Autodesk Inventor part; units mm, degrees
ref_plane "YZ Plane" through (0, 0, 0) normal (1, 0, 0) x (0, 1, 0)
ref_plane "XZ Plane" through (0, 0, 0) normal (0, 1, 0) x (-1, 0, 0)
ref_plane "XY Plane" through (0, 0, 0) normal (0, 0, 1) x (1, 0, 0)
sketch "Sketch1" plane through (0, 0, 0) normal (0, 0, 1) x (1, 0, 0)
  spline S0 degree 3 poles (-8.9262, 55.5372) (-8.7839, 55.3802) (-8.4991, 55.0662) (-8.0852, 54.5835) (-7.6813, 54.0924) (-7.2889, 53.592) (-6.9084, 53.0826) (-6.5406, 52.5638) (-6.1865, 52.0357) (-5.8469, 51.4981) (-5.5231, 50.9508) (-5.2164, 50.3937) (-4.9286, 49.8267) (-4.6617, 49.2495) (-4.4187, 48.6617) (-4.2033, 48.0633) (-4.0539, 47.5547) (-3.9553, 47.1422) (-3.9241, 46.9325) (-3.9085, 46.8277) knots 0 0 0 0 0.063581 0.127162 0.190743 0.254324 0.317905 0.381486 0.445066 0.508647 0.572227 0.635807 0.699386 0.762964 0.826542 0.890117 0.953687 0.985476 1.017256 1.017256 1.017256 1.017256
  spline S1 degree 3 poles (-3.9085, 46.8277) (-3.8988, 46.6849) (-3.8795, 46.3993) (-3.8286, 45.9728) (-3.7545, 45.5498) (-3.6583, 45.1311) (-3.5319, 44.7205) (-3.3763, 44.3201) (-3.189, 43.9333) (-2.9645, 43.5666) (-2.7433, 43.2845) (-2.5493, 43.0739) (-2.3922, 42.9274) (-2.2262, 42.7911) (-2.0526, 42.6646) (-1.8686, 42.5537) (-1.678, 42.4548) (-1.4812, 42.3683) (-1.2769, 42.302) (-1.0697, 42.2449) (-0.8577, 42.21) (-0.6441, 42.187) (-0.3577, 42.1846) (0, 42.1894) (0.3577, 42.1846) (0.6441, 42.187) (0.8577, 42.21) (1.0697, 42.2449) (1.2769, 42.302) (1.4812, 42.3683) (1.678, 42.4548) (1.8686, 42.5537) (2.0526, 42.6646) (2.2262, 42.7911) (2.3922, 42.9274) (2.5493, 43.0739) (2.7433, 43.2845) (2.9645, 43.5666) (3.189, 43.9333) (3.3763, 44.3201) (3.5319, 44.7205) (3.6583, 45.1311) (3.7545, 45.5498) (3.8286, 45.9728) (3.8795, 46.3993) (3.8988, 46.6849) (3.9085, 46.8277) knots 0 0 0 0 0.04293 0.085861 0.12879 0.17172 0.214646 0.257562 0.300476 0.343394 0.386302 0.407769 0.429238 0.450698 0.472163 0.49363 0.515088 0.536554 0.558017 0.579478 0.600945 0.622403 0.64387 0.686802 0.729734 0.751201 0.772659 0.794126 0.815587 0.83705 0.858516 0.879974 0.901441 0.922906 0.944366 0.965835 0.987302 1.03021 1.073128 1.116042 1.158958 1.201884 1.244814 1.287743 1.330674 1.373604 1.373604 1.373604 1.373604
  spline S2 degree 3 poles (3.9085, 46.8277) (3.9241, 46.9325) (3.9553, 47.1422) (4.0539, 47.5547) (4.2033, 48.0633) (4.4187, 48.6617) (4.6617, 49.2495) (4.9286, 49.8267) (5.2164, 50.3937) (5.5231, 50.9508) (5.8469, 51.4981) (6.1865, 52.0357) (6.5406, 52.5638) (6.9084, 53.0826) (7.2889, 53.592) (7.6813, 54.0924) (8.0852, 54.5835) (8.4991, 55.0662) (8.7839, 55.3802) (8.9262, 55.5372) knots 0 0 0 0 0.03178 0.063568 0.127139 0.190714 0.254291 0.31787 0.381449 0.445029 0.508609 0.572189 0.63577 0.699351 0.762932 0.826513 0.890094 0.953675 1.017256 1.017256 1.017256 1.017256
  circle A0 centre (0, 0) radius 42.1875 construction
  circle A1 centre (0, 0) radius 46.9846 construction
  circle A2 centre (0, 0) radius 50 construction
  circle A3 centre (0, 0) radius 56.25
  point P0 (-8.5013, 55.0643)
  point P1 (-8.0869, 54.5821)
  point P2 (-7.6832, 54.0908)
  point P3 (-7.2909, 53.5905)
  point P4 (-6.9105, 53.081)
  point P5 (-6.5429, 52.5623)
  point P6 (-6.1889, 52.0341)
  point P7 (-5.8496, 51.4965)
  point P8 (-5.526, 50.9492)
  point P9 (-5.2196, 50.3921)
  point P10 (-4.9321, 49.825)
  point P11 (-4.6657, 49.2477)
  point P12 (-4.4233, 48.6599)
  point P13 (-4.2093, 48.0613)
  point P14 (-4.031, 47.4511)
  point P15 (-3.9598, 47.1413)
  point P16 (-3.8758, 46.3996)
  point P17 (-3.8247, 45.9733)
  point P18 (-3.7508, 45.5505)
  point P19 (-3.6533, 45.1324)
  point P20 (-3.527, 44.7221)
  point P21 (-3.371, 44.3223)
  point P22 (-3.1828, 43.9367)
  point P23 (-2.9576, 43.5713)
  point P24 (-2.6935, 43.2332)
  point P25 (-2.5474, 43.0758)
  point P26 (-2.3907, 42.9291)
  point P27 (-2.225, 42.7928)
  point P28 (-2.0509, 42.6672)
  point P29 (-1.8675, 42.5557)
  point P30 (-1.677, 42.4569)
  point P31 (-1.48, 42.3717)
  point P32 (-1.2764, 42.3036)
  point P33 (-1.069, 42.2486)
  point P34 (-0.8574, 42.212)
  point P35 (-0.6439, 42.1905)
  point P36 (-0.4293, 42.1857)
  point P37 (0, 42.1875)
  point P38 (0.4293, 42.1857)
  point P39 (0.6439, 42.1905)
  point P40 (0.8574, 42.212)
  point P41 (1.069, 42.2486)
  point P42 (1.2764, 42.3036)
  point P43 (1.48, 42.3717)
  point P44 (1.677, 42.4569)
  point P45 (1.8675, 42.5557)
  point P46 (2.0509, 42.6672)
  point P47 (2.225, 42.7928)
  point P48 (2.3907, 42.9291)
  point P49 (2.5474, 43.0758)
  point P50 (2.6935, 43.2332)
  point P51 (2.9576, 43.5713)
  point P52 (3.1828, 43.9367)
  point P53 (3.371, 44.3223)
  point P54 (3.527, 44.7221)
  point P55 (3.6533, 45.1324)
  point P56 (3.7508, 45.5505)
  point P57 (3.8247, 45.9733)
  point P58 (3.8758, 46.3996)
  point P59 (3.9598, 47.1413)
  point P60 (4.031, 47.4511)
  point P61 (4.2093, 48.0613)
  point P62 (4.4233, 48.6599)
  point P63 (4.6657, 49.2477)
  point P64 (4.9321, 49.825)
  point P65 (5.2196, 50.3921)
  point P66 (5.526, 50.9492)
  point P67 (5.8496, 51.4965)
  point P68 (6.1889, 52.0341)
  point P69 (6.5429, 52.5623)
  point P70 (6.9105, 53.081)
  point P71 (7.2909, 53.5905)
  point P72 (7.6832, 54.0908)
  point P73 (8.0869, 54.5821)
  point P74 (8.5013, 55.0643)
extrude "Extrusion1" add sketch "Sketch1" against normal blind 16
extrude "Extrusion2" cut sketch "Sketch1" against normal through all contours A3 S2 S1 S0 picked at (0.9155, 51.5438)
pattern_circular "Circular Pattern1" count 16 over 360 about axis through (0, 0, 0) along (0, 0, -1) of "Extrusion2"
sketch "Measuring" plane through (0, 0, -16) normal (0, 0, -1) x (-1, 0, 0)
  circle A0 centre (0, 0) radius 56.25
  circle A1 centre (0, 0) radius 50
  circle A2 centre (73.063, 68.2774) radius 50 construction
  line L0 (27.9744, 52.4494) -> (54.2214, 24.3627) construction
  line L1 (41.0979, 38.406) -> (73.063, 68.2774) construction
  dimension "d37" = 100
  dimension "d45" = 6.25
  dimension "d46" = 100
  dimension "d47" = 43.75
sketch "Sketch11" plane through (0, 0, 0) normal (1, 0, 0) x (0, 1, 0)
  line L0 (13.8864, 0) -> (-13.8864, 0) construction
  line L1 (-13.8864, 0) -> (-13.8864, -7) construction
  line L2 (-13.8864, -7) -> (13.8864, -7) construction
  line L3 (13.8864, -7) -> (13.8864, 0) construction
  circle A0 centre (0, -3.5) radius 1.5 construction
  line L4 (-1.3941, -2) -> (1.3941, -2) construction
  line L5 (-3.9085, -16) -> (3.9085, -16) construction
  line L6 (-67.1444, 3.8787) -> (73.9482, 3.8787)
  line L7 (73.9482, 3.8787) -> (73.9482, -7)
  line L8 (73.9482, -7) -> (-67.1444, -7)
  line L9 (-67.1444, -7) -> (-67.1444, 3.8787)
  point P0 (0, 0)
  point P1 (0, 0)
  point P2 (-13.8864, -3.5)
  point P3 (0, -2)
  dimension "d48" = 3
  dimension "d49" = 2
  dimension "d50" = 9
  dimension "d58" = 7
extrude "Thinner" cut sketch "Sketch11" against normal through all both and the other way through all
sketch "Sketch12" plane through (-16.8651, 41.399, -7) normal (0, 0, 1) x (0.9476, 0.3195, 0)
  circle A0 centre (2.7546, -44.6175) radius 3
  dimension "d54" = 6
extrude "Hole" cut sketch "Sketch12" against normal blind 20
sketch "Sketch13" plane through (-16.8651, 41.399, -7) normal (0, 0, 1) x (0.9476, 0.3195, 0)
  circle A0 centre (2.7546, -44.6175) radius 11
  circle A1 centre (2.7546, -44.6175) radius 3
  dimension "d57" = 8
extrude "Coupler" add sketch "Sketch13" along normal blind 7
sketch "Sketch14" plane through (-16.8651, 41.399, -7) normal (0, 0, 1) x (0.9476, 0.3195, 0)
  circle A0 centre (11.251, -19.4175) radius 9
  line L0 (16.2331, -4.641) -> (2.7546, -44.6175) construction
  circle A1 centre (2.7546, -44.6175) radius 11 construction
  circle A2 centre (2.7546, -44.6175) radius 11 construction
  line L1 (6.269, -34.194) -> (16.2331, -4.641) construction
  circle A3 centre (-14.821, -24.6594) radius 9
  circle A4 centre (-23.3174, -49.8593) radius 9
  circle A5 centre (-5.7418, -69.8174) radius 9
  circle A6 centre (20.3302, -64.5756) radius 9
  circle A7 centre (28.8266, -39.3756) radius 9
  dimension "d61" = 18
  dimension "d64" = 360
extrude "Cutouts" cut sketch "Sketch14" against normal through all
sketch "Sketch15" plane through (0, 0, 0) normal (1, 0, 0) x (0, 1, 0)
  circle A0 centre (0, -3.5) radius 1.5
  line L0 (11, 0) -> (-11, 0)
  line L1 (0, 0) -> (0, -7) construction
  line L2 (0, -7) -> (0, 0) construction
  line L3 (-11, -7) -> (11, -7) construction
  point P0 (0, 0)
  point P1 (-10.9663, -7)
  dimension "d68" = 3
extrude "SetScrewHole1" cut sketch "Sketch15" along normal through all
sketch "Sketch16" plane through (0, 0, 0) normal (0, 1, 0) x (-1, 0, 0)
  circle A0 centre (0, -3.5) radius 1.5
  line L0 (-11, -7) -> (11, -7)
  line L1 (0, 0) -> (0, -7) construction
  dimension "d71" = 3
extrude "Extrusion14" cut sketch "Sketch16" along normal through all
thread "Thread3"
thread "Thread4"
sketch "Sketch17" plane through (-16.8651, 41.399, -7) normal (0, 0, 1) x (0.9476, 0.3195, 0)
  line L0 (-62.2572, 14.3784) -> (64.742, 14.3784)
  line L1 (64.742, 14.3784) -> (64.742, -104.7192)
  line L2 (64.742, -104.7192) -> (-62.2572, -104.7192)
  line L3 (-62.2572, -104.7192) -> (-62.2572, 14.3784)
  point P0 (2.7546, -44.6175)
extrude "Extrusion15" cut sketch "Sketch17" against normal blind 10
sketch "Sketch18" plane through (0, 0, -7) normal (0, 0, -1) x (-1, 0, 0)
  circle A0 centre (0, 0) radius 50
  dimension "d80" = 100
extrude "Extrusion16" add sketch "Sketch18" along normal blind 3
sketch "Sketch19" plane through (0, 0, -10) normal (0, 0, -1) x (-1, 0, 0)
  line L0 (-50, 50) -> (50, 50) construction
  line L1 (50, 50) -> (50, -50) construction
  line L2 (50, -50) -> (-50, -50) construction
  line L3 (-50, -50) -> (-50, 50) construction
  circle A0 centre (0, 0) radius 50
sketch "Sketch20" plane through (0, 0, 0) normal (1, 0, 0) x (0, 1, 0)
  line L0 (-50, -7) -> (50, -7)
  line L1 (18.4735, 2.9106) -> (10, 2.9106)
  line L2 (10, 2.9106) -> (10, -7)
  line L3 (10, -7) -> (18.4735, -7)
  line L4 (18.4735, -7) -> (18.4735, 2.9106)
  point P0 (0, 0)
  dimension "d124" = 10
extrude "Extrusion17" cut sketch "Sketch20" along normal through all both and the other way through all
equation "\"Module\" = 6.25"
equation "\"PressureAngle\" = 20deg"
equation "\"UnitProfileClearance\" = 0.25"
equation "\"UnitRoundRadius\" = 0.35"
equation "\"HeadDiameter\" = 112.5"
equation "\"RootDiameter\" = 84.375"
equation "\"BaseDiameter\" = 93.96926"
equation "\"HelixAngle\" = 0"
equation "\"UnitCorrection\" = 0"
equation "\"UnitAddendumModification\" = 0"
equation "\"CircularPitch\" = 19.634954"
equation "\"UnitBacklashShift\" = 0"
equation "\"TotalToolShift\" = 0"
equation "\"IsInternal\" = 0"
properties part number "wheel"
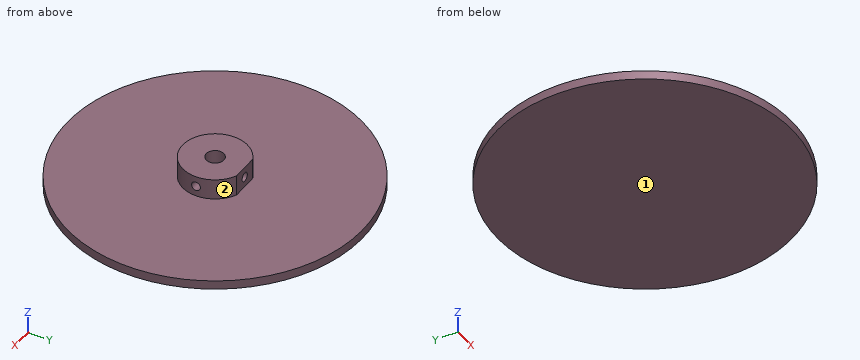
The listing builds one solid part. Answer for the finished solid, in the listing's coordinates (mm). Face numbers are marked on the shaded views. A direction names the side the tool comes from. Round coordinates to 2 decimals unless told otherwise and drop trailing zeros. Order: outer loops, then holes, each group sorted by start corner. A loop starts at its lowest first (then second) coordinate and runs counter-clockwise, first axis right, second up. Notation, with made-up numbers: M -12,46.25 L 41,46.25 A13 ccw 41,57.25 Z; hole C 67.25,-31 d9. An arc over 180 degrees is marked long. Answer in a Markdown table with one row per item. Add a question column.
1) Consider line 1 along Z through (x, y) = (0, 8); line 2 along Z through (x, y) = (-21.5, 11.5); line 3 along X through (y, z) = (5.25, -3.5). Determine where each line is inside the solid, lowest interval first. Write a range as from..to.
2) The part is cut by section B-B on z = -3.5. Determine the outline of the cut face in (x, y), plus the area to 3 significant figures.
3) The part is cut by section A-A on x = 0. Determine the outline of the cut face in (y, z).
4) Which of the six approach directions +Z, -Z, +X, -X, +Y, -Y give full straight-line access (tool end or side, diameter ignored) to the marked faces 1 and 2?
5) The part is cut by section C-C on y = 13. Determine the outline of the cut face in (x, z).
6) The part is cut by section D-D on x = -20.5. Determine the outline of the cut face in (y, z).
7) Flat-ended cylindrical pins translate along their axes: pin 1 Ø3.5 at (y, z) = (0, -3.5) entering from -X; pin 2 Ø2 at (x, z) = (0, -2.5) entering from +Y; pin 3 Ø3 at (x, z) = (29, -8.5) entering from -Y. Find the tip coordinate at first contact, or state that the pin passes through.
Findings below:
| question | item | result |
|---|---|---|
| 1 | line 1 | z = -10..-5, -2..0 |
| 1 | line 2 | z = -10..-7 |
| 1 | line 3 | x = -9.67..-1.5, 1.5..9.67 |
| 2 | outline | M -4.58,10 A11 ccw long 10.9,-1.5 L 2.6,-1.5 A3 cw long -1.5,2.6 L -1.5,10 Z; M 1.5,2.6 A3 cw 2.6,1.5 L 10.9,1.5 A11 ccw 4.58,10 L 1.5,10 Z |
| 2 | area | 300 mm² |
| 3 | outline | M -50,-10 L 50,-10 L 50,-7 L 10,-7 L 10,-5 L 3,-5 L 3,-7 L -3,-7 L -3,0 L -11,0 L -11,-7 L -50,-7 Z; M 3,-2 L 10,-2 L 10,0 L 3,0 Z |
| 4 | face 1 | -Z, +X, -X, +Y, -Y |
| 4 | face 2 | +Z |
| 5 | outline | M -48.28,-10 L 48.28,-10 L 48.28,-7 L -48.28,-7 Z |
| 6 | outline | M -45.6,-10 L 45.6,-10 L 45.6,-7 L -45.6,-7 Z |
| 7 | pin 1 | stops at x = -11 |
| 7 | pin 2 | stops at y = 10 |
| 7 | pin 3 | stops at y = -41.76 |
